```python
from build123d import *

# Parameters (mm, degrees)
SKETCH1_R           = 2.5
BOSS_EXTRUDE1_DEPTH = 2.286
CUT_EXTRUDE1_DEPTH  = 823.59169598
FILLET1_R           = 5.08


with BuildPart() as part:
    # Sketch1 → Boss-Extrude1 (new body)
    with BuildSketch(Plane.XY):
        with BuildLine():
            Line((-7.62, 755.65), (210.82, 755.65))
            ThreePointArc((210.82, 755.65), (214.412102448, 757.137897552), (215.9, 760.73))
            Line((215.9, 760.73), (215.9, 788.67))
            ThreePointArc((215.9, 788.67), (214.412102448, 792.262102448), (210.82, 793.75))
            Line((210.82, 793.75), (-7.62, 793.75))
            ThreePointArc((-7.62, 793.75), (-11.212102448, 792.262102448), (-12.7, 788.67))
            Line((-12.7, 788.67), (-12.7, 760.73))
            ThreePointArc((-12.7, 760.73), (-11.212102448, 757.137897552), (-7.62, 755.65))
        make_face()
        with Locations((0, 762)):
            Circle(SKETCH1_R, mode=Mode.SUBTRACT)
        with Locations((0, 774.7)):
            Circle(SKETCH1_R, mode=Mode.SUBTRACT)
        with Locations((0, 787.4)):
            Circle(SKETCH1_R, mode=Mode.SUBTRACT)
        with Locations((203.2, 762)):
            Circle(SKETCH1_R, mode=Mode.SUBTRACT)
        with Locations((203.2, 774.7)):
            Circle(SKETCH1_R, mode=Mode.SUBTRACT)
        with Locations((203.2, 787.4)):
            Circle(SKETCH1_R, mode=Mode.SUBTRACT)
        with BuildLine():
            Line((17.78, 783.59), (79.760886363, 783.59))
            ThreePointArc((79.760886363, 783.59), (81.075687113, 783.416903198), (82.300886363, 782.909409051))
            Line((82.300886363, 782.909409051), (95.499113517, 775.289409051))
            ThreePointArc((95.499113517, 775.289409051), (97.866016715, 769.575199251), (92.959113517, 765.81))
            Line((92.959113517, 765.81), (17.78, 765.81))
            ThreePointArc((17.78, 765.81), (14.187897552, 767.297897552), (12.7, 770.89))
            Line((12.7, 770.89), (12.7, 778.51))
            ThreePointArc((12.7, 778.51), (14.187897552, 782.102102448), (17.78, 783.59))
        make_face(mode=Mode.SUBTRACT)
        with BuildLine():
            Line((190.5, 778.51), (190.5, 770.89))
            ThreePointArc((190.5, 770.89), (189.012102448, 767.297897552), (185.42, 765.81))
            Line((185.42, 765.81), (123.439113517, 765.81))
            ThreePointArc((123.439113517, 765.81), (122.124312768, 765.983096802), (120.899113517, 766.490590949))
            Line((120.899113517, 766.490590949), (107.700886363, 774.110590949))
            ThreePointArc((107.700886363, 774.110590949), (105.333983166, 779.824800749), (110.240886363, 783.59))
            Line((110.240886363, 783.59), (185.42, 783.59))
            ThreePointArc((185.42, 783.59), (189.012102448, 782.102102448), (190.5, 778.51))
        make_face(mode=Mode.SUBTRACT)
    extrude(amount=BOSS_EXTRUDE1_DEPTH)

    # Sketch3 → Cut-Extrude1 (cut, through all)
    with BuildSketch(Plane(origin=(0, 0, 0), x_dir=(-1, 0, 0), z_dir=(0, 0, -1))):
        with BuildLine():
            Line((-210.82, 755.65), (-208.28, 755.65))
            Line((-208.28, 755.65), (-208.28, 793.75))
            Line((-208.28, 793.75), (-210.82, 793.75))
            ThreePointArc((-210.82, 793.75), (-214.412102448, 792.262102448), (-215.9, 788.67))
            Line((-215.9, 788.67), (-215.9, 760.73))
            ThreePointArc((-215.9, 760.73), (-214.412102448, 757.137897552), (-210.82, 755.65))
        make_face()
        with BuildLine():
            Line((5.08, 793.75), (5.08, 755.65))
            Line((5.08, 755.65), (7.62, 755.65))
            ThreePointArc((7.62, 755.65), (11.212102448, 757.137897552), (12.7, 760.73))
            Line((12.7, 760.73), (12.7, 788.67))
            ThreePointArc((12.7, 788.67), (11.212102448, 792.262102448), (7.62, 793.75))
            Line((7.62, 793.75), (5.08, 793.75))
        make_face()
    extrude(amount=-CUT_EXTRUDE1_DEPTH, mode=Mode.SUBTRACT)

    # Fillet1
    fillet1_edges = [part.edges().sort_by_distance(p)[0] for p in [
        (208.28, 755.65, 1.143),
        (208.28, 793.75, 1.143),
        (-5.08, 755.65, 1.143),
        (-5.08, 793.75, 1.143),
    ]]
    fillet(fillet1_edges, radius=FILLET1_R)


solid = part.part
```
Work out the finished part from the listing and answer in its coordinate system (mm). A direction names the side the tool comes from. Round coordinates to 2 decimals unless told otherwise and drop trailing zeros. Write each loop counter-clockwise with the first axis right and the second up, starting at its lowest first coordinate (ties: lowest second). Pieces come first, ordered by that corner, then holes. Notation, with made-up numbers: (-5, 21) - (22, 21) arc R22 ccw to (22, 38) - close; hole circle Ø8 at (78, 11). An arc over 180 degrees is marked (long way). Return JSON: item names as keys, results as strings. Group by question number.
Q1. This flat-tipped pin is pushed along its axis until it touches: pin 1 Ø1.5 at (x, y) = (119, 781) entering from +Z. Where does it stop, or does it pass through?
Q2. The part is cut by section A-A on z = 1.35. Count the separate pieces of the cut face and the enclosed holes in it, then the cut area to 3 significant figures.
Q3. The mould has two halves that part along Y. Classify faces 1 (the cylindrical face through (206.752, 757.099, 1.159)), 2 (the cylindrical face through (105.31, 779.73, 1.13)), 3 (the flat face through (100, 775, 0)), 4 (the flat face through (114.39, 770.25, 1.13)): released by +Y, released by -Y, zero draft, split by the parting line, or undercut.
Q4. For faces 5 (the cylindrical face through (206.831, 792.222, 1.159)), 6 (the cylindrical face through (14.149, 782.062, 1.127)), determine the directions among +Z, -Z, +X, -X, +Y, -Y from which every point of the face is accessible in a straight line to the end or side of a thin tool.
Q5. Find the intervals of material crossed by L1, parallel to X at y = 762, z = 0.8; L2, parallel to Y at x = 203.2, z = 1.45; L3, parallel to Y at x = 29, z = 1.85, in increasing order.
Q6. The part is cut by section B-B on x = 68. Write down the section's boundary in (y, z).
Solved:
{
 "1": {"pin 1": "through"},
 "2": {"separate pieces": "1", "enclosed holes": "8", "area": "5,160 mm²"},
 "3": {"face 1": "released by -Y", "face 2": "undercut", "face 3": "zero draft", "face 4": "undercut"},
 "4": {"face 5": "+Z, -Z, +X, +Y", "face 6": "+Z, -Z"},
 "5": {"L1": "-5.08 to -2.5, 2.5 to 200.7, 205.7 to 208.28", "L2": "755.65 to 759.5, 764.5 to 772.2, 777.2 to 784.9, 789.9 to 793.75", "L3": "755.65 to 765.81, 783.59 to 793.75"},
 "6": {"outline": "(755.65, 0) - (765.81, 0) - (765.81, 2.29) - (755.65, 2.29) - close; (783.59, 0) - (793.75, 0) - (793.75, 2.29) - (783.59, 2.29) - close"}
}
